```python
from build123d import *

# Parameters (mm, degrees)
BOSS_EXTRUDE1_DEPTH                             = 25
CUT_EXTRUDE1_DEPTH                              = 21
CUT_EXTRUDE1_DEPTH_BACK                         = 21
SKETCH2_W                                       = 40
SKETCH2_H                                       = 42
CUT_EXTRUDE2_DEPTH                              = 69.300805266
CUT_EXTRUDE2_DEPTH_BACK                         = 69.300805266
SKETCH3_R                                       = 11.25
SKETCH4_R                                       = 11.25
SKETCH4_R_2                                     = 9.75
BOSS_EXTRUDE2_DEPTH                             = 2
TAP_DRILL_FOR_M3X0_5_TAP1_D                     = 2.5
CSK_FOR_M3_FLAT_HEAD_MACHINE_SCREW1_D           = 3.2
CSK_FOR_M3_FLAT_HEAD_MACHINE_SCREW1_DEPTH       = 10
CSK_FOR_M3_FLAT_HEAD_MACHINE_SCREW1_CSINK_D     = 6.3
CSK_FOR_M3_FLAT_HEAD_MACHINE_SCREW1_CSINK_ANGLE = 90
CSK_FOR_M3_FLAT_HEAD_MACHINE_SCREW2_D           = 3.2
CSK_FOR_M3_FLAT_HEAD_MACHINE_SCREW2_CSINK_D     = 6.3
CSK_FOR_M3_FLAT_HEAD_MACHINE_SCREW2_CSINK_ANGLE = 90
CHAMFER1_SIZE                                   = 0.5
BOSS_EXTRUDE3_START                             = -44
SKETCH4_2_R                                     = 11.25
SKETCH4_2_R_2                                   = 9.75
BOSS_EXTRUDE3_DEPTH                             = 4


with BuildPart() as part:
    # Sketch1 → Boss-Extrude1 (new, symmetric)
    with BuildSketch(Plane.XY):
        Polygon((-10, 21), (-10, -11), (-20, -21), (-30, -21), (-50, -1), (-50, 21), (-58, 21), (-58, -26), (42, -26), (42, -21), (0, 21), align=None)
    extrude(amount=BOSS_EXTRUDE1_DEPTH, both=True)

    # Sketch2 → Cut-Extrude1 (cut, two sides: drawn at the far end of the back side and taken through both)
    with BuildSketch(Plane.XY.offset(-CUT_EXTRUDE1_DEPTH_BACK)):
        with Locations((-30, 0)):
            Rectangle(SKETCH2_W, SKETCH2_H)
        Polygon((0, 21), (0, -21), (42, -21), align=None)
    extrude(amount=CUT_EXTRUDE1_DEPTH + CUT_EXTRUDE1_DEPTH_BACK, mode=Mode.SUBTRACT)

    # Sketch3 → Cut-Extrude2 (cut, two sides: drawn at the far end of the back side and taken through both)
    with BuildSketch(Plane(origin=(0, 0, 0), x_dir=(0, 0, -1), z_dir=(1, 0, 0)).offset(-CUT_EXTRUDE2_DEPTH_BACK)):
        Circle(SKETCH3_R)
    extrude(amount=CUT_EXTRUDE2_DEPTH + CUT_EXTRUDE2_DEPTH_BACK, mode=Mode.SUBTRACT)

    # Sketch4 → Boss-Extrude2 (add)
    with BuildSketch(Plane.ZY.offset(50)):
        with Locations(Location((0, 0, 0), (0, 0, 180))):
            Circle(SKETCH4_R)
        with Locations(Location((0, 0, 0), (0, 0, 270))):
            Circle(SKETCH4_R_2, mode=Mode.SUBTRACT)
    extrude(amount=BOSS_EXTRUDE2_DEPTH)

    # Tap Drill for M3x0.5 Tap1 (through all)
    with Locations(Plane.ZY.offset(58)):
        with Locations((-9.545941546, 9.545941546), (9.545941546, -9.545941546)):
            Hole(TAP_DRILL_FOR_M3X0_5_TAP1_D / 2)

    # CSK for M3 Flat Head Machine Screw1
    with Locations(Plane.ZY.offset(10)):
        with Locations((-16, 16), (16, 16), (16, -16), (-16, -16), (0, 0)):
            CounterSinkHole(CSK_FOR_M3_FLAT_HEAD_MACHINE_SCREW1_D / 2, CSK_FOR_M3_FLAT_HEAD_MACHINE_SCREW1_CSINK_D / 2, depth=CSK_FOR_M3_FLAT_HEAD_MACHINE_SCREW1_DEPTH, counter_sink_angle=CSK_FOR_M3_FLAT_HEAD_MACHINE_SCREW1_CSINK_ANGLE)

    # CSK for M3 Flat Head Machine Screw2 (through all)
    with Locations(Plane(origin=(0, -21, 0), x_dir=(1, 0, 0), z_dir=(0, 1, 0))):
        with Locations((-44, 15), (-16, 15), (36, 15), (36, -15), (-16, -15), (-44, -15), (6, -15), (6, 15)):
            CounterSinkHole(CSK_FOR_M3_FLAT_HEAD_MACHINE_SCREW2_D / 2, CSK_FOR_M3_FLAT_HEAD_MACHINE_SCREW2_CSINK_D / 2, counter_sink_angle=CSK_FOR_M3_FLAT_HEAD_MACHINE_SCREW2_CSINK_ANGLE)

    # Chamfer1
    chamfer1_edges = [part.edges().sort_by_distance(p)[0] for p in [
        (0, 0, 11.25),
        (-58, 0, 11.25),
        (-10, -16, -21),
        (-10, -16, 21),
        (-15, -21, 21),
        (-10, -21, 0),
        (-15, -21, -21),
        (-50, -11, 21),
        (-50, -11, -21),
        (-40, -21, -21),
        (-50, -21, 0),
        (-40, -21, 21),
        (21, -21, 21),
        (0, -21, 0),
        (21, -21, -21),
        (0, 21, 0),
        (-10, 21, 0),
        (-5, 21, 25),
        (-10, 5, 25),
        (-15, -16, 25),
        (-25, -21, 25),
        (-40, -11, 25),
        (-50, 10, 25),
        (-54, 21, 25),
        (-50, 21, 0),
        (-58, 21, 0),
        (-54, 21, -25),
        (-50, 10, -25),
        (-40, -11, -25),
        (-25, -21, -25),
        (-15, -16, -25),
        (-10, 5, -25),
        (-5, 21, -25),
        (21, 0, 25),
        (21, 0, -25),
        (42, -23.5, 25),
        (42, -23.5, -25),
        (-58, -2.5, -25),
        (-58, -2.5, 25),
        (42, -26, 0),
        (-8, -26, -25),
        (-58, -26, 0),
        (-8, -26, 25),
    ]]
    chamfer(chamfer1_edges, length=CHAMFER1_SIZE)

    # Sketch4<2> → Boss-Extrude3 (add)
    with BuildSketch(Plane.ZY.offset(50).offset(BOSS_EXTRUDE3_START)):
        with Locations(Location((0, 0, 0), (0, 0, 180))):
            Circle(SKETCH4_2_R)
        with Locations(Location((0, 0, 0), (0, 0, 270))):
            Circle(SKETCH4_2_R_2, mode=Mode.SUBTRACT)
    extrude(amount=BOSS_EXTRUDE3_DEPTH)


solid = part.part
```
Design review of the part built by this model. Coordinates are the model's own, in mm. A direction names the side the tool comes from. Coordinates: 2 decimals unless noted, no trailing zeros. Order: outer loops, then holes, each group sorted by start corner. A loop starts at its lowest first (then second) coordinate and runs counter-clockwise, first axis right, second up. Notation, with made-up numbers: (28.25, -27) -> (80.25, -27) arc R23 cw to (80.25, -7) -> close; hole circle Ø11 at (-8, 84.5). An arc over 180 degrees is marked (long way). One line per item, written item: value. Start each with the question number.
Q1. Take a section at B-B, the plane z = 0. Give the number of separate pieces and of enclosed holes in the cut face, then the cut area to 3 significant figures.
Q2. Insertion check: pin 1 Ø20.5 at (x, z) = (22.5, 10) entering from +Y; pin 2 Ø12.5 at (y, z) = (-8.5, 8.5) entering from +X; pin 3 Ø6 at (x, y) = (-18.5, -11.5) entering from -Z; pin 4 Ø4 at (x, z) = (36, 15) entering from +Y. Each pin has a flat end and moves straight along its axis. Give the tip position at first contact, or say it passes through.
Q3. Tool access review of faces 3 (the flat face through (-30, -21, 0)), 4 (the flat face through (16, -4, 21)), 5 (the cylindrical face through (36.208, -24.299, -16.586)), 6 (the flat face through (-58, -12, 0)), 7 (the cylindrical face through (-4.17, -15.93, -14.4)): name each direction out of +Z, -Z, +X, -X, +Y, -Y from which nothing blocks a thin tool from reaching the whole face with its end or side.
Q4. For probe 1 along Z at (x, y) = (-44, -23); probe 2 along X at (y, z) = (-12, -9.5); probe 3 along X at (y, z) = (-25.1, 15), list the stretches that pass through material, from the lowest coordinate up.
Q5. Mouldability with a two-part tool opening along Z and no side actions: class faces 1 (the flat face through (-40, -11, 23)), 2 (the flat face through (-6, -10, 0)) as pulls with the +Z half, pulls with the -Z half, needs draft (parallel to the pull), parting line crosses it, or undercut.
Q6. Take a section at A-A, the plane x = 6. State the section outline as (y, z) points, then the cut area to 3 significant figures.
Q7. Take a section at C-C, the plane x = 36. State the section outline as (y, z) points, then the cut area to 3 significant figures.
Values follow:
1. separate pieces: 3
1. enclosed holes: 0
1. area: 868 mm2
2. pin 1: stops at y = -21
2. pin 2: stops at x = 0
2. pin 3: passes through
2. pin 4: stops at y = -22.15
3. face 3: +Y
3. face 4: +X, +Y
3. face 5: +Y, -Y
3. face 6: +Z, -Z, -X, +Y, -Y
3. face 7: +X
4. probe 1: z = -25 to -16.6, -13.4 to 13.4, 16.6 to 25
4. probe 2: x = -58 to -50, -10 to 0
4. probe 3: x = -58 to -45.6, -42.4 to -17.6, -14.4 to 4.4, 7.6 to 34.4, 37.6 to 42
5. face 1: needs draft
5. face 2: undercut
6. outline: (-26, -24.5) -> (-25.5, -25) -> (14.29, -25) -> (15, -24.5) -> (15, -21) -> (-20.5, -21) -> (-21, -20.5) -> (-21, -18.15) -> (-22.55, -16.6) -> (-26, -16.6) -> close; (-26, -13.4) -> (-22.55, -13.4) -> (-21, -11.85) -> (-21, 11.85) -> (-22.55, 13.4) -> (-26, 13.4) -> close; (-26, 16.6) -> (-22.55, 16.6) -> (-21, 18.15) -> (-21, 20.5) -> (-20.5, 21) -> (15, 21) -> (15, 24.5) -> (14.29, 25) -> (-25.5, 25) -> (-26, 24.5) -> close
6. area: 501 mm2
7. outline: (-26, -24.5) -> (-25.5, -25) -> (-15.71, -25) -> (-15, -24.5) -> (-15, -21) -> (-20.5, -21) -> (-21, -20.5) -> (-21, -18.15) -> (-22.55, -16.6) -> (-26, -16.6) -> close; (-26, -13.4) -> (-22.55, -13.4) -> (-21, -11.85) -> (-21, 11.85) -> (-22.55, 13.4) -> (-26, 13.4) -> close; (-26, 16.6) -> (-22.55, 16.6) -> (-21, 18.15) -> (-21, 20.5) -> (-20.5, 21) -> (-15, 21) -> (-15, 24.5) -> (-15.71, 25) -> (-25.5, 25) -> (-26, 24.5) -> close
7. area: 261 mm2
